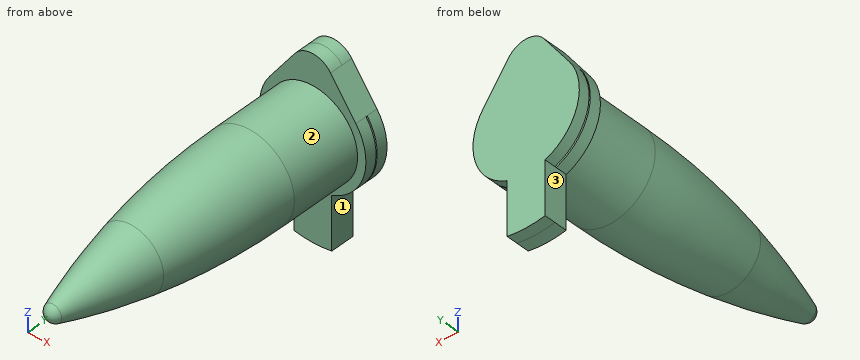
Autodesk Inventor part; units mm, degrees
ref_plane "YZ Plane" through (0, 0, 0) normal (1, 0, 0) x (0, 1, 0)
ref_plane "XZ Plane" through (0, 0, 0) normal (0, 1, 0) x (-1, 0, 0)
ref_plane "XY Plane" through (0, 0, 0) normal (0, 0, 1) x (1, 0, 0)
sketch "Sketch1" plane through (0, 0, 0) normal (0, 0, 1) x (1, 0, 0)
  line L0 (3, 15.24) -> (3, 20)
  line L1 (3, 20) -> (2.7, 20)
  line L2 (2.7, 20) -> (2.7, 13.7288)
  line L3 (0, 0.6837) -> (0, 0)
  arc A0 (0, 0) -> (0.5935, 0.4276) centre (0, 0.6256) ccw
  arc A1 (0.5935, 0.4276) -> (3, 15.24) centre (-43.7889, 15.24) ccw
  line L4 (0, 0) -> (-1.9294, 0)
  arc A2 (0, 0.6837) -> (0.5584, 1.3498) centre (-0.6188, 1.7696) ccw
  arc A3 (0.5584, 1.3498) -> (2.7, 13.7288) centre (-34.1481, 13.7288) ccw
  line L5 (-6.5051, 6.35) -> (10.1936, 6.35)
  line L6 (2.1819, 6.35) -> (2.1819, 2.9816)
  dimension "d0" = 3
  dimension "d1" = 15.24
  dimension "d2" = 20
  dimension "d3" = 2.7
  dimension "d7" = 6.35
  dimension "d8" = 2.1819
revolve "Revolution1" add sketch "Sketch1" angle 360 about axis through (0, 0.6837, 0) along (0, -1, 0)
sketch "Sketch2" plane through (0, 20, 0) normal (0, 1, 0) x (1, 0, 0)
  circle A0 centre (0, 0) radius 3.556
  circle A1 centre (0, 0) radius 2.7
  dimension "d9" = 7.112
extrude "Extrusion1" add sketch "Sketch2" along normal blind 0.762
sketch "Sketch3" plane through (0, 0, 0) normal (1, 0, 0) x (0, 1, 0)
  line L0 (21.5893, 0) -> (20.8527, 0)
  line L1 (20.8527, 0) -> (20.8527, -6.985)
  line L2 (20.8527, -6.985) -> (21.5893, -6.985)
  line L3 (21.5893, -6.985) -> (21.5893, 0)
  line L4 (20.762, -3.556) -> (20.762, 3.556)
  line L5 (20, 3.556) -> (20, -3.556)
  line L6 (20.8527, -2.6155) -> (20, -2.6155)
  line L7 (20, -2.6155) -> (20, -1.9879)
  line L8 (20, -1.9879) -> (20.8527, -1.9879)
  line L9 (20.8527, -1.9879) -> (20.8527, -2.6155)
  point P0 (0, 0)
  point P1 (20.762, 0)
  dimension "d12" = 6.985
  dimension "d13" = 0.7366
revolve "Revolution2" add sketch "Sketch3" angle 360 about axis through (0, 21.5893, 0) along (0, -1, 0)
sketch "Sketch4" plane through (0, 21.5893, 0) normal (0, 1, 0) x (1, 0, 0)
  line L0 (-1.1941, -4.4189) -> (-2.8822, -2.0828)
  circle A0 centre (0, 0) radius 3.556
  line L1 (2.8822, -2.0828) -> (1.1941, -4.4189)
  line L2 (1.27, 3.3215) -> (1.27, 6.8686)
  circle A1 centre (0, 0) radius 6.985
  line L3 (-1.27, 3.3215) -> (-1.27, 6.8686)
  line L4 (-1.27, 6.8686) -> (1.27, 6.8686)
  circle A2 centre (0, 0) radius 3.556
  arc A3 (-1.1941, -4.4189) -> (1.1941, -4.4189) centre (0, -3.556) ccw
  line L5 (0, -5.0292) -> (-1.1247, -5.0292)
  point P0 (0, 6.8686)
  dimension "d15" = 2.54
  dimension "d16" = 5.0292
extrude "Extrusion2" cut sketch "Sketch4" against normal blind 25.4 contours A3 L1 A0 L2 A1 L3 L0
sketch "Sketch5" plane through (0, 20.8527, 3.556) normal (0, -1, 0) x (1, 0, 0)
  circle A0 centre (0, -3.556) radius 3.556
  circle A1 centre (0, -3.556) radius 2.6155
  line L0 (1.27, -10.4246) -> (1.27, -6.8775)
  arc A2 (1.27, -6.8775) -> (2.8822, -1.4732) centre (0, -3.556) ccw
  line L1 (2.8822, -1.4732) -> (1.1941, 0.8629)
  arc A3 (1.1941, 0.8629) -> (-1.1941, 0.8629) centre (0, 0) ccw
  line L2 (-1.1941, 0.8629) -> (-2.8822, -1.4732)
  arc A4 (-2.8822, -1.4732) -> (-1.27, -6.8775) centre (0, -3.556) ccw
  line L3 (-1.27, -6.8775) -> (-1.27, -10.4246)
  arc A5 (-1.27, -10.4246) -> (1.27, -10.4246) centre (0, -3.556) ccw
extrude "Extrusion3" add sketch "Sketch5" along normal up to surface (0.8527 mm away) contours A0 L2 A3 L1 | L0 A5 L3 A0
properties part number "Vial" material "Glass"
Input: part model. Units: mm. Frame: model coordinates. Face numbers are marked on the shaded views. A direction names the side the tool comes from. Give positions to 0.01 mm unless a question says otherwise; leave off trailing zeros. Loops run counter-clockwise (first coordinate to the right, second up) from the corner with the lowest first, then second, coordinate; pieces in that order, holes last. Notation, with made-up numbers: (68, -18.75) -> (118, -18.75) arc R17 cw to (118, 7.25) -> close; hole circle Ø2 at (-37, 24.5). An arc over 180 degrees is marked (long way). Use a Markdown table: item, result.
Q1. Ray query, probe 1 along Z at (x, y) = (0, 16.25); probe 2 along Y at (x, z) = (0.75, -5.25); probe 3 along X at (y, z) = (8.75, 0.5). Return the intervals inside material, ascending. Write a range as from..to.
Entries:
| item | result |
|---|---|
| probe 1 | z = -3..-2.7, 2.7..3 |
| probe 2 | y = 20..21.59 |
| probe 3 | x = -2.5..-2.31, 2.31..2.5 |
Q2. Section query C-C, the plane z = -4. Return the cut outline in (x, y).
Entries:
| item | result |
|---|---|
| outline | (-1.27, 20) -> (1.27, 20) -> (1.27, 21.59) -> (-1.27, 21.59) -> close |
Q3. Section query A-A, the plane y = 18.5. Return the cut outline in (x, z), plus the area to 3 significant figures.
Entries:
| item | result |
|---|---|
| outline | circle Ø6 at (0, 0); hole circle Ø5.4 at (0, 0) |
| area | 5.37 mm² |
Q4. First-contact query: P1, Ø3.5, axis at x = 1, z = 1.5, coming from the -Y side; P2, Ø2.5, axis at x = -1.5, z = -0.5, coming from the -Y side; P3, Ø0.8, axis at y = 21, z = -5.5, coming from the +X side. Flat tips, straight axial feed; report the tip coordinate or a pass-through.
Entries:
| item | result |
|---|---|
| P1 | stops at y = 0 |
| P2 | stops at y = 0.09 |
| P3 | stops at x = 1.27 |
Q5. Access query for the marked faces 1, 2 and 3. Directions: +Z, -Z, +X, -X, +Y, -Y. A direction counts if a zero-diameter tool reaches every point of the face in a straight line with its end or side. Return the directions, or none.
Entries:
| item | result |
|---|---|
| face 1 | -Z, +X, +Y, -Y |
| face 2 | -Y |
| face 3 | -Z, -X, +Y, -Y |
Q6. Section query B-B, the plane z = 4. Return the cut outline in (x, y), plus the area to 3 significant figures.
Entries:
| item | result |
|---|---|
| outline | (-1.5, 20) -> (1.5, 20) -> (1.5, 21.59) -> (-1.5, 21.59) -> close |
| area | 4.76 mm² |
